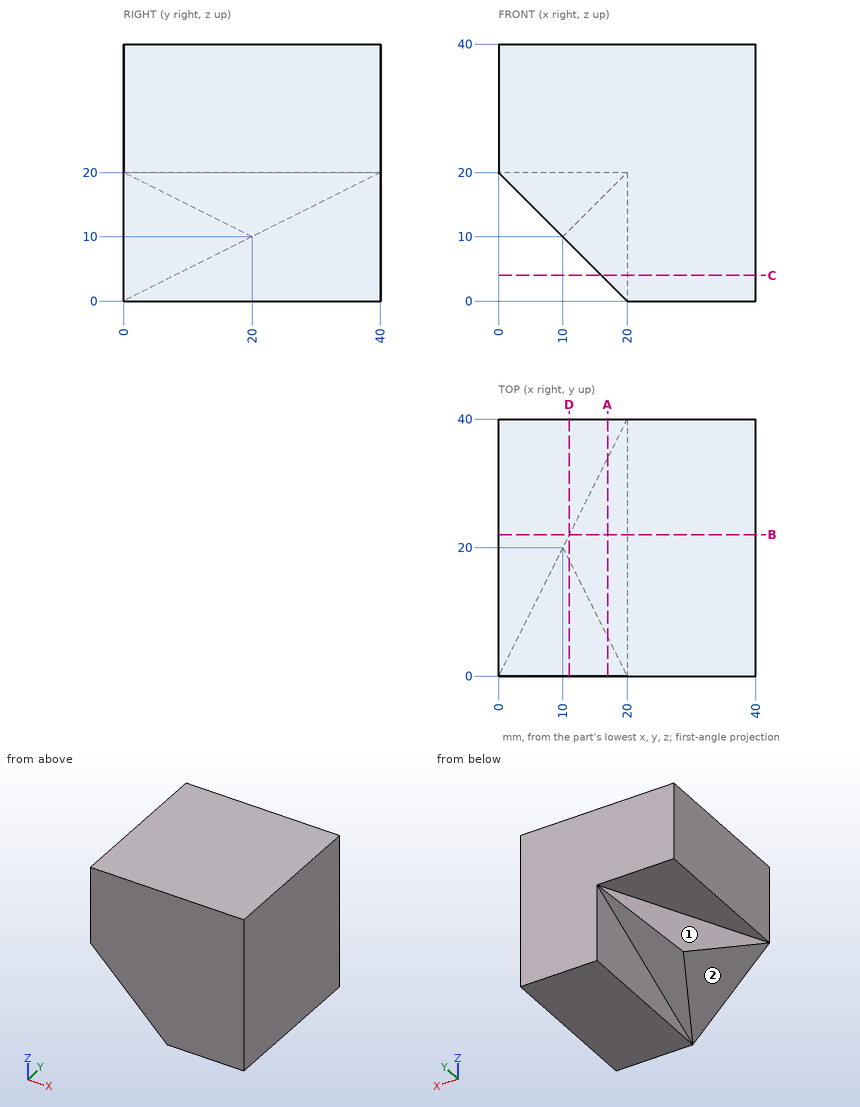
Drawing for the job (mm, zero at the part's lowest x, y, z). A direction names the side the tool comes from. Give positions to 0.01 mm unless a question says otherwise; leave off trailing zeros. Write each loop counter-clockwise with the first axis right and the second up, starting at its lowest first coordinate (ties: lowest second). Pieces come first, ordered by that corner, then holes. Notation, with made-up numbers: (25, 44) -> (76, 44) arc R16 cw to (76, 64) -> close; hole circle Ø9 at (-16.75, 19). An arc over 180 degrees is marked (long way). Put each result on its own line as item: value. Start each with the question number.
Item 1: Pin check, flat tips, straight feed: pin 1 Ø8 at (x, y) = (13.5, 23) entering from -Z; pin 2 Ø6 at (y, z) = (17.5, 10.5) entering from -X. Stop position of each tip, or through.
Item 2: Wall check: L1, parallel to X at y = 33, z = 5; L2, parallel to X at y = 24, z = 18; L3, parallel to Y at x = 16.5, z = 7. Give the ranges that are in metal, low to high. Write a range as [from, to].
Item 3: Cut at A-A (x = 17). List the corners of the cut face in (y, z), then the cut area to 3 significant figures.
Item 4: Cut at C-C (z = 4). List the corners of the cut face in (x, y).
Item 5: Cut at B-B (y = 22). List the corners of the cut face in (x, z), then the cut area to 3 significant figures.
Item 6: Cut at D-D (x = 11). List the corners of the cut face in (y, z), then the cut area to 3 significant figures.
Item 7: Which spindle directions (+Z, -Z, +X, -X, +Y, -Y) get a long thin tool onto all of the face, cutting with end or side? Do the marked faces 1 and 2. Say none if no direction does.
Answer list:
1. pin 1: stops at z = 9.5
1. pin 2: stops at x = 7.59
2. L1: x = [20, 40]
2. L2: x = [12, 40]
2. L3: y = [0, 14]
3. outline: (0, 3) -> (6, 3) -> (34, 17) -> (34, 20) -> (40, 20) -> (40, 40) -> (0, 40) -> close
3. area: 1,180 mm2
4. outline: (16, 0) -> (40, 0) -> (40, 40) -> (20, 40) -> (20, 8) -> (16, 8) -> close
5. outline: (0, 20) -> (11, 20) -> (11, 11) -> (20, 11) -> (20, 0) -> (40, 0) -> (40, 40) -> (0, 40) -> close
5. area: 1,280 mm2
6. outline: (0, 9) -> (18, 9) -> (22, 11) -> (22, 20) -> (40, 20) -> (40, 40) -> (0, 40) -> close
6. area: 1,040 mm2
7. face 1: -Z, -X, +Y
7. face 2: -Z, -X, +Y, -Y
